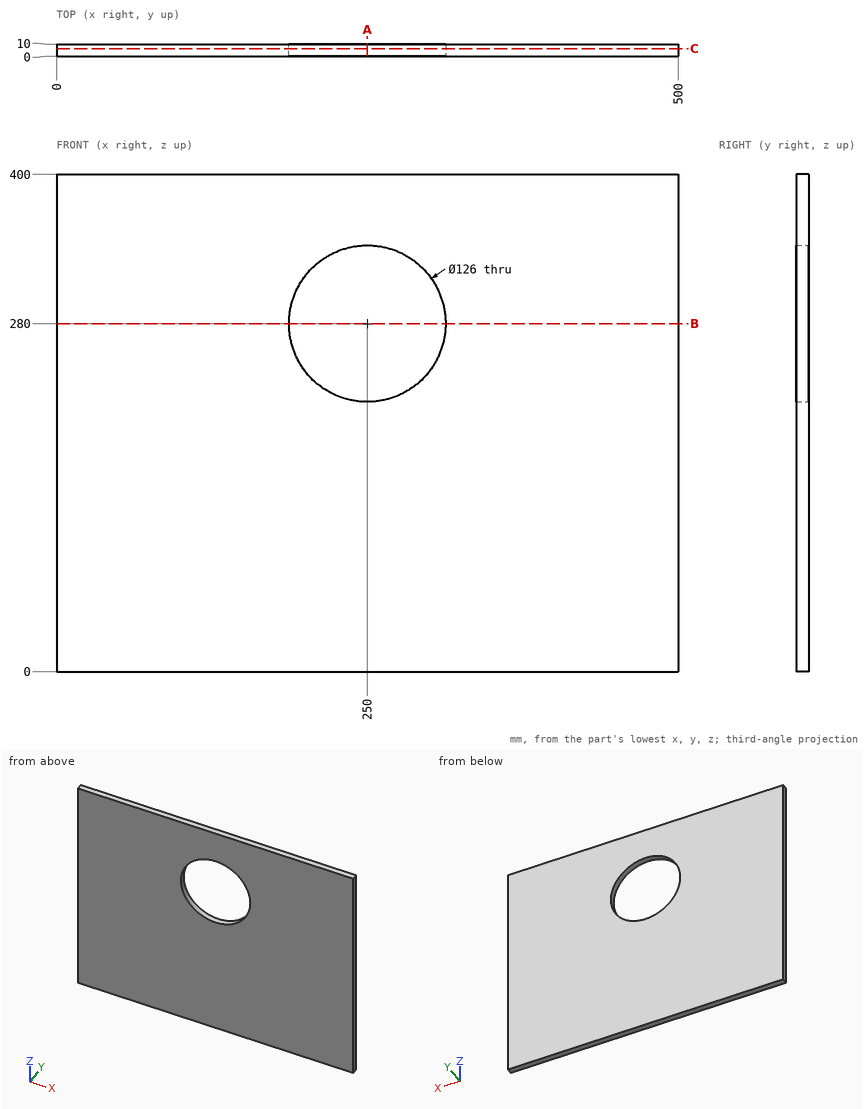
Check sheet for the drawn part. Datum: minimum x, y, z corner. Units: mm. Round coordinates to 2 decimals unless told otherwise and drop trailing zeros. Order: outer loops, then holes, each group sorted by start corner. A loop starts at its lowest first (then second) coordinate and runs counter-clockwise, first axis right, second up. Notation, with made-up numbers: (26, -19.5) -> (77, -19.5) arc R25 ccw to (77, 8.5) -> close; hole circle Ø9 at (3, 1.25). An arc over 180 degrees is marked (long way). Return JSON: item names as keys, results as strings. Group by question number.
Q1. Section check B-B, the plane z = 280. Record the boundary of the cut face in (x, y).
Q2. Section check C-C, the plane y = 6.25. Record the boundary of the cut face in (x, z), plus the area to 3 significant figures.
Q3. Material ranges on probe 1 along Z at (x, y) = (250, 7.5); probe 2 along X at (y, z) = (6, 280); probe 3 along X at (y, z) = (6.25, 301.5), recorded low to high. Write a range as from..to.
Q4. Gauge pin test, flat end, axial feed: pin 1 (4 mm diameter, centred on x = 179, z = 296.5, fed in from -Y). Record the tip position at first contact, or that the pin passes through.
Q5. Section check A-A, the plane x = 250. Record the boundary of the cut face in (y, z), plus the area to 3 significant figures.
Numbers:
{
 "1": {"outline": "(0, 0) -> (187, 0) -> (187, 10) -> (0, 10) -> close; (313, 0) -> (500, 0) -> (500, 10) -> (313, 10) -> close"},
 "2": {"outline": "(0, 0) -> (500, 0) -> (500, 400) -> (0, 400) -> close; hole circle Ø126 at (250, 280)", "area": "188,000 mm^2"},
 "3": {"probe 1": "0..217, 343..400", "probe 2": "0..187, 313..500", "probe 3": "0..190.78, 309.22..500"},
 "4": {"pin 1": "y = 0"},
 "5": {"outline": "(0, 0) -> (10, 0) -> (10, 217) -> (0, 217) -> close; (0, 343) -> (10, 343) -> (10, 400) -> (0, 400) -> close", "area": "2,740 mm^2"}
}
